```python
from build123d import *

# Parameters (mm, degrees)
F0_W     = 23.876
F0_H     = 15.748
F1_DEPTH = 3.20802
F3_T     = -1.778
F4_R     = 3.2385
F4_R_2   = 2.6416
F5_DEPTH = 3.06898


# Not quite as in the source:
# - a feature names something its author has since deleted; it is built from what else it names


with BuildPart() as f1:
    # F0 (on Top) → F1 (new body)
    with BuildSketch(Plane.XY):
        with Locations((11.938, 7.874)):
            Rectangle(F0_W, F0_H)
    extrude(amount=F1_DEPTH)

    # F3
    f3_openings = [f1.faces().sort_by_distance(p)[0] for p in [
        (11.938, 7.874, 0),
    ]]
    offset(amount=F3_T, openings=f3_openings)

    # F4 (on face) → F5 (join)
    with BuildSketch(Plane.XY):
        with BuildLine():
            ThreePointArc((4.1275, 7.5388690457), (7.366, 4.3003690457), (10.6045, 7.5388690457))
            ThreePointArc((10.6045, 7.5388690457), (7.366, 10.7773690457), (4.1275, 7.5388690457))
        make_face()
        with BuildLine():
            ThreePointArc((10.0076, 7.5388690457), (7.366, 4.8972690457), (4.7244, 7.5388690457))
            ThreePointArc((4.7244, 7.5388690457), (7.366, 10.1804690457), (10.0076, 7.5388690457))
        make_face(mode=Mode.SUBTRACT)
        with Locations((15.24, 7.5388690457)):
            Circle(F4_R)
        with Locations((15.24, 7.5388690457)):
            Circle(F4_R_2, mode=Mode.SUBTRACT)
    extrude(amount=F5_DEPTH)


solid = f1.part
```
Build history of the part. All positions in model axes, mm. A direction names the side the tool comes from. Give positions to 0.01 mm unless a question says otherwise; leave off trailing zeros. Loops run counter-clockwise (first coordinate to the right, second up) from the corner with the lowest first, then second, coordinate; pieces in that order, holes last. Notation, with made-up numbers: (6, -9.5) -> (20, -9.5) arc R21 ccw to (20, 7.5) -> close; hole circle Ø11 at (53.5, -10.75). An arc over 180 degrees is marked (long way). One line per question, with ' | ' between items. Start each with the question number.
1) Cut at D-D (x = 2.5). Give the cut face in (y, z).
2) Two-plate mould, pull along Y, no slides. Class faces 3 (the cylindrical face through (12.005, 7.681, 0.705)), 4 (the flat face through (1.778, 8, 1)), 5 (the flat face through (12, 8, 3.208)), 6 (the flat face through (12, 15.748, 2)): released by +Y, released by -Y, zero draft, split by the parting line, or undercut.
3) Pin check, flat tips, straight feed: pin 1 (1 mm diameter, centred on y = 4, z = 2, fed in from -X); pin 2 (1.6 mm diameter, centred on x = 7.5, y = 7.5, fed in from -Z). Stop position of each tip, or through.
4) Cut at A-A (z = 0.85). Give the cut face in (x, y).
5) 3-axis set-ups, long thin cutter, end or side, ignore diameter. For faces 1 (the cylindrical face through (10.005, 7.655, 0.705)), 2 (the flat face through (12, 1, 0)): which of +Z, -Z, +X, -X, +Y, -Y reach the whole face in a straight line?
6) Cut at C-C (y = 4). Give the cut face in (x, z).
7) Probe L1, parallel to Y at x = 15.24, z = 1; L2, parallel to X at y = 7.5, z = 1.15; L3, parallel to Y at x = 5.5, z = 0.8. List the from-to ranges inside material, lowest first.
8) Cut at B-B (x = 15.24). Give the cut face in (y, z).
Return value:
1) outline: (0, 0) -> (1.78, 0) -> (1.78, 1.43) -> (13.97, 1.43) -> (13.97, 0) -> (15.75, 0) -> (15.75, 3.21) -> (0, 3.21) -> close
2) face 3: undercut | face 4: undercut | face 5: zero draft | face 6: released by +Y
3) pin 1: x = 0 | pin 2: z = 1.43
4) outline: (0, 0) -> (23.88, 0) -> (23.88, 15.75) -> (0, 15.75) -> close; circle Ø6.48 at (7.37, 7.54); circle Ø6.48 at (15.24, 7.54); hole (1.78, 1.78) -> (22.1, 1.78) -> (22.1, 13.97) -> (1.78, 13.97) -> close; hole circle Ø5.28 at (7.37, 7.54); hole circle Ø5.28 at (15.24, 7.54)
5) face 1: -Z | face 2: -Z, +X, -X, +Y, -Y
6) outline: (0, 0) -> (1.78, 0) -> (1.78, 1.43) -> (22.1, 1.43) -> (22.1, 0) -> (23.88, 0) -> (23.88, 3.21) -> (0, 3.21) -> close
7) L1: 0 to 1.78, 4.3 to 4.9, 10.18 to 10.78, 13.97 to 15.75 | L2: 0 to 1.78, 4.13 to 4.72, 10.01 to 10.6, 12 to 12.6, 17.88 to 18.48, 22.1 to 23.88 | L3: 0 to 1.78, 4.89 to 5.67, 9.41 to 10.19, 13.97 to 15.75
8) outline: (0, 0) -> (1.78, 0) -> (1.78, 1.43) -> (4.3, 1.43) -> (4.3, 0) -> (4.9, 0) -> (4.9, 1.43) -> (10.18, 1.43) -> (10.18, 0) -> (10.78, 0) -> (10.78, 1.43) -> (13.97, 1.43) -> (13.97, 0) -> (15.75, 0) -> (15.75, 3.21) -> (0, 3.21) -> close
